```python
from build123d import *

# Parameters (mm, degrees)
SKETCH_1_R          = 1.5
EXTRUDE_1_DEPTH     = 3
EXTRUDE_2_DEPTH     = 10
SKETCH_7_R          = 1.25
CUT_EXTRUDE_7_DEPTH = 32.701734968
CUT_EXTRUDE_8_DEPTH = 31.935416597


with BuildPart() as part:
    # 草图1 → 凸台-拉伸1 (new body)
    with BuildSketch(Plane(origin=(0, 0, 0), x_dir=(1, 0, 0), z_dir=(0, 1, 0))):
        with BuildLine():
            Line((0, 3), (26, 3))
            ThreePointArc((26, 3), (29, 0), (26, -3))
            Line((26, -3), (0, -3))
            ThreePointArc((0, -3), (-3, 0), (0, 3))
        make_face()
        with Locations(Location((0, 0, 0), (0, 0, 270))):
            Circle(SKETCH_1_R, mode=Mode.SUBTRACT)
        with Locations(Location((26, 0, 0), (0, 0, 270))):
            Circle(SKETCH_1_R, mode=Mode.SUBTRACT)
    extrude(amount=EXTRUDE_1_DEPTH)

    # 草图6 → 凸台-拉伸2 (add)
    with BuildSketch(Plane.XZ):
        with BuildLine():
            Line((10.5, 4), (15.5, 4))
            ThreePointArc((15.5, 4), (19.5, 0), (15.5, -4))
            Line((15.5, -4), (10.5, -4))
            ThreePointArc((10.5, -4), (6.5, 0), (10.5, 4))
        make_face()
    extrude(amount=-EXTRUDE_2_DEPTH)

    # 草图7 → 切除-拉伸7 (cut, through all)
    with BuildSketch(Plane(origin=(0, 0, -4), x_dir=(-1, 0, 0), z_dir=(0, 0, -1))):
        with Locations((-13, 7)):
            Circle(SKETCH_7_R)
    extrude(amount=-CUT_EXTRUDE_7_DEPTH, mode=Mode.SUBTRACT)

    # 草图9 → 切除-拉伸8 (cut, through all)
    with BuildSketch(Plane(origin=(0, 10, 0), x_dir=(1, 0, 0), z_dir=(0, 1, 0))):
        with BuildLine():
            Line((10.5, -2), (15.5, -2))
            ThreePointArc((15.5, -2), (17.5, 0), (15.5, 2))
            Line((15.5, 2), (10.5, 2))
            ThreePointArc((10.5, 2), (8.5, 0), (10.5, -2))
        make_face()
    extrude(amount=-CUT_EXTRUDE_8_DEPTH, mode=Mode.SUBTRACT)


solid = part.part
```
Design review of the part built by this model. Coordinates are the model's own, in mm. A direction names the side the tool comes from. Coordinates: 2 decimals unless noted, no trailing zeros. Loops run counter-clockwise (first coordinate to the right, second up) from the corner with the lowest first, then second, coordinate; pieces in that order, holes last. Notation, with made-up numbers: M 76.25,74.25 L 108.25,74.25 A14 ccw 108.25,100.25 Z; hole C -33.5,79.25 d3. An arc over 180 degrees is marked long. One line per question, with ' | ' between items.
(1) We need section A-A (x = 13). Give the boundary of the cut face in (y, z), and give its area (3 significant figures).
Filled in:
outline: M 0,-4 L 5.75,-4 L 5.75,-2 L 0,-2 Z; M 0,2 L 5.75,2 L 5.75,4 L 0,4 Z; M 8.25,-4 L 10,-4 L 10,-2 L 8.25,-2 Z; M 8.25,2 L 10,2 L 10,4 L 8.25,4 Z | area: 30.0 mm^2
(2) Wall thickness on probe 1 along X at (y, z) = (1.1, 0); probe 2 along Z at (x, y) = (14, 9.75); probe 3 along Y at (x, z) = (13, -3.2): over which ranges is each line inside the solid? List them lowest first.
Filled in:
probe 1: x = -3 to -1.5, 1.5 to 8.5, 17.5 to 24.5, 27.5 to 29 | probe 2: z = -4 to -2, 2 to 4 | probe 3: y = 0 to 5.75, 8.25 to 10
(3) We need section D-D (y = 6.25). Give the boundary of the cut face in (x, z).
Filled in:
outline: M 10.5,-4 L 12,-4 L 12,-2 L 10.5,-2 A2 cw 10.5,2 L 12,2 L 12,4 L 10.5,4 A4 ccw Z; M 14,-4 L 15.5,-4 A4 ccw 15.5,4 L 14,4 L 14,2 L 15.5,2 A2 cw 15.5,-2 L 14,-2 Z
(4) For pin 1 Ø1.5 at (x, y) = (21, 8) entering from +Z; pin 2 Ø3.5 at (x, y) = (24, 1) entering from -Z; pin 3 Ø1.5 at (y, z) = (5.5, -0.5) entering from +X; pin 4 Ø4 at (y, z) = (2, 3) entering from +X, all flat-tipped, find the tip position at first contact; note any pin that passes through.
Filled in:
pin 1: passes through | pin 2: stops at z = -3 | pin 3: stops at x = 19.5 | pin 4: stops at x = 28.83
(5) Draft analysis for pull direction Z (two halves, no side actions). For faces 4 (the face through (22, 1, -3)), 5 (the face through (13, 5, -2)), 6 (the face through (24, 3, 0)), state which applies: released by +Z, released by -Z, zero draft, split by the parting line, or undercut.
Filled in:
face 4: released by -Z | face 5: undercut | face 6: zero draft
(6) We need section B-B (y = 1.5). Give the boundary of the cut face in (x, z).
Filled in:
outline: M 0,-3 L 7.85,-3 A4 ccw 10.5,-4 L 15.5,-4 A4 ccw 18.15,-3 L 26,-3 A3 ccw 26,3 L 18.15,3 A4 ccw 15.5,4 L 10.5,4 A4 ccw 7.85,3 L 0,3 A3 ccw Z; hole C 0,0 d3; hole M 10.5,-2 L 15.5,-2 A2 ccw 15.5,2 L 10.5,2 A2 ccw Z; hole C 26,0 d3
(7) We need section C-C (z = 0). Give the boundary of the cut face in (x, y), and give its area (3 significant figures).
Filled in:
outline: M -3,0 L -1.5,0 L -1.5,3 L -3,3 Z; M 1.5,0 L 8.5,0 L 8.5,10 L 6.5,10 L 6.5,3 L 1.5,3 Z; M 17.5,0 L 24.5,0 L 24.5,3 L 19.5,3 L 19.5,10 L 17.5,10 Z; M 27.5,0 L 29,0 L 29,3 L 27.5,3 Z | area: 79.0 mm^2
(8) Machinability: for faces 1 (the face through (4, 1, -3)), 2 (the face through (4, 1, 3)), 3 (the face through (17.5, 5.1, 0)), which of the approach directions +Z, -Z, +X, -X, +Y, -Y give a long, thin tool a straight path to every point of the face, cutting with its end or side? Answer none if there is none.
Filled in:
face 1: -Z, -X, +Y, -Y | face 2: +Z, -X, +Y, -Y | face 3: +Y, -Y
